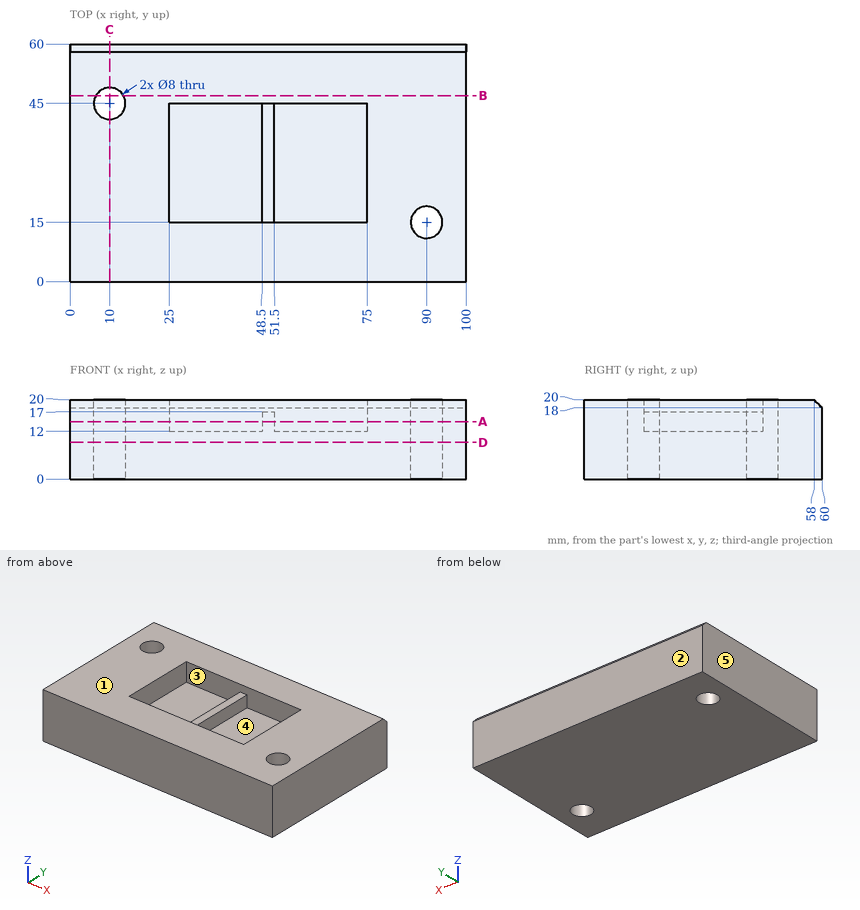
Verification items for this drawing (mm, ordinates from the low corner). A direction names the side the tool comes from. Coordinates: 2 decimals unless noted, no trailing zeros. Write each loop counter-clockwise with the first axis right and the second up, starting at its lowest first coordinate (ties: lowest second). Pieces come first, ordered by that corner, then holes. Notation, with made-up numbers: M 32,37 L 63,37 A16 cw 63,44 Z; hole C -28,82 d10. An arc over 180 degrees is marked long. Answer as a JSON object with one key per item and string values.
1. Scan lines: L1, parallel to X at y = 37, z = 15; L2, parallel to X at y = 35.5, z = 18.75; L3, parallel to Y at x = 90, z = 15. Record each from-to range of solid material in increasing order.
Answers below:
{"L1": "x = 0 to 25, 48.5 to 51.5, 75 to 100", "L2": "x = 0 to 25, 75 to 100", "L3": "y = 0 to 11, 19 to 60"}
2. Section check D-D, the plane z = 9.25. Enter the section's corners in (x, y), plus the area to 3 significant figures.
Answers below:
{"outline": "M 0,0 L 100,0 L 100,60 L 0,60 Z; hole C 10,45 d8; hole C 90,15 d8", "area": "5,900 mm²"}
3. Section check C-C, the plane x = 10. Enter the section's corners in (y, z), plus the area to 3 significant figures.
Answers below:
{"outline": "M 0,0 L 41,0 L 41,20 L 0,20 Z; M 49,0 L 60,0 L 60,18 L 58,20 L 49,20 Z", "area": "1,040 mm²"}
4. Draft check along Y on the marked faces 1, 2 and 3. Enter one of: released by +Y, released by -Y, zero draft, split by the parting line, or undercut.
Answers below:
{"face 1": "zero draft", "face 2": "released by +Y", "face 3": "undercut"}
5. Tool access check on the marked faces 4 and 5. Record the directions out of +Z, -Z, +X, -X, +Y, -Y that give a thin tool (end or side, any length) a straight path to the whole face; none if there is none.
Answers below:
{"face 4": "+Z", "face 5": "+Z, -Z, -X, +Y, -Y"}
6. Go/stop test with flat-tipped pins: pin 1 Ø7 at (x, y) = (36, 24) entering from +Z; pin 2 Ø3.5 at (x, y) = (49.5, 24) entering from +Z. Record where each tip stops, or that it passes through.
Answers below:
{"pin 1": "stops at z = 12", "pin 2": "stops at z = 17"}
7. Section check A-A, the plane z = 14.5. Enter the section's corners in (x, y), plus the area to 3 significant figures.
Answers below:
{"outline": "M 0,0 L 100,0 L 100,60 L 0,60 Z; hole C 10,45 d8; hole M 25,15 L 48.5,15 L 48.5,45 L 25,45 Z; hole M 51.5,15 L 75,15 L 75,45 L 51.5,45 Z; hole C 90,15 d8", "area": "4,490 mm²"}
8. Section check B-B, the plane y = 47. Enter the section's corners in (x, z), plus the area to 3 significant figures.
Answers below:
{"outline": "M 0,0 L 6.54,0 L 6.54,20 L 0,20 Z; M 13.46,0 L 100,0 L 100,20 L 13.46,20 Z", "area": "1,860 mm²"}
